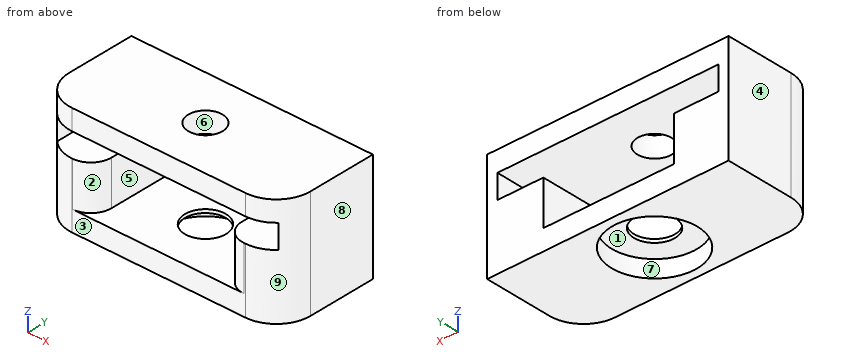
from build123d import *

# Parameters (mm, degrees)
SKETCH1_W           = 70.659898478
SKETCH1_H           = 30
BOSS_EXTRUDE1_DEPTH = 6
SKETCH2_R           = 5
CUT_EXTRUDE1_DEPTH  = 10
FILLET1_R           = 10
BOSS_EXTRUDE2_DEPTH = 7
BOSS_EXTRUDE3_DEPTH = 13
FILLET2_R           = 6
BOSS_EXTRUDE4_DEPTH = 6
SKETCH8_R           = 6
CUT_EXTRUDE2_DEPTH  = 30
SKETCH9_R           = 12.5
CUT_EXTRUDE3_DEPTH  = 5


with BuildPart() as part:
    # Sketch1 → Boss-Extrude1 (new body)
    with BuildSketch(Plane.XY):
        Rectangle(SKETCH1_W, SKETCH1_H)
    extrude(amount=BOSS_EXTRUDE1_DEPTH)

    # Sketch2 → Cut-Extrude1 (cut)
    with BuildSketch(Plane(origin=(0, 0, 0), x_dir=(-1, 0, 0), z_dir=(0, 0, -1))):
        Circle(SKETCH2_R)
    extrude(amount=-CUT_EXTRUDE1_DEPTH, mode=Mode.SUBTRACT)

    # Fillet1
    fillet1_edges = [part.edges().sort_by_distance(p)[0] for p in [
        (35.329949239, -15, 3),
        (-35.329949239, -15, 3),
    ]]
    fillet(fillet1_edges, radius=FILLET1_R)

    # Sketch4 → Boss-Extrude2 (add)
    with BuildSketch(Plane(origin=(0, 0, 0), x_dir=(-1, 0, 0), z_dir=(0, 0, -1))):
        with BuildLine():
            Line((-32.40101705, -12.071067812), (-32.316998846, 15))
            Line((-32.316998846, 15), (-35.329949239, 15))
            Line((-35.329949239, 15), (-35.329949239, -5))
            ThreePointArc((-35.329949239, -5), (-34.568744564, -8.826834324), (-32.40101705, -12.071067812))
        make_face()
        with BuildLine():
            Line((35.329949239, -5), (35.329949239, 15))
            Line((35.329949239, 15), (32.40101705, 15))
            Line((32.40101705, 15), (32.40101705, -12.071067812))
            ThreePointArc((32.40101705, -12.071067812), (34.568744564, -8.826834324), (35.329949239, -5))
        make_face()
    extrude(amount=BOSS_EXTRUDE2_DEPTH)

    # Sketch6 → Boss-Extrude3 (add)
    with BuildSketch(Plane(origin=(0, 0, -7), x_dir=(-1, 0, 0), z_dir=(0, 0, -1))):
        with BuildLine():
            Line((-18.889389891, 15), (-18.889389891, -15))
            Line((-18.889389891, -15), (-25.329949239, -15))
            ThreePointArc((-25.329949239, -15), (-32.40101705, -12.071067812), (-35.329949239, -5))
            Line((-35.329949239, -5), (-35.329949239, 15))
            Line((-35.329949239, 15), (-18.889389891, 15))
        make_face()
        with BuildLine():
            Line((19.317805732, 15), (19.317805732, -15))
            Line((19.317805732, -15), (25.329949239, -15))
            ThreePointArc((25.329949239, -15), (32.40101705, -12.071067812), (35.329949239, -5))
            Line((35.329949239, -5), (35.329949239, 15))
            Line((35.329949239, 15), (19.317805732, 15))
        make_face()
    extrude(amount=BOSS_EXTRUDE3_DEPTH)

    # Fillet2
    fillet2_edges = [part.edges().sort_by_distance(p)[0] for p in [
        (-19.317805732, -15, -13.5),
        (18.889389891, -15, -13.5),
    ]]
    fillet(fillet2_edges, radius=FILLET2_R)

    # Sketch7 → Boss-Extrude4 (add)
    with BuildSketch(Plane(origin=(0, 0, -20), x_dir=(-1, 0, 0), z_dir=(0, 0, -1))):
        with BuildLine():
            Line((-25.329949239, -15), (25.329949239, -15))
            ThreePointArc((25.329949239, -15), (32.40101705, -12.071067812), (35.329949239, -5))
            Line((35.329949239, -5), (35.329949239, 15))
            Line((35.329949239, 15), (-35.329949239, 15))
            Line((-35.329949239, 15), (-35.329949239, -5))
            ThreePointArc((-35.329949239, -5), (-32.40101705, -12.071067812), (-25.329949239, -15))
        make_face()
    extrude(amount=BOSS_EXTRUDE4_DEPTH)

    # Sketch8 → Cut-Extrude2 (cut)
    with BuildSketch(Plane.XY.offset(-20)):
        Circle(SKETCH8_R)
    extrude(amount=-CUT_EXTRUDE2_DEPTH, mode=Mode.SUBTRACT)

    # Sketch9 → Cut-Extrude3 (cut)
    with BuildSketch(Plane(origin=(0, 0, -26), x_dir=(-1, 0, 0), z_dir=(0, 0, -1))):
        Circle(SKETCH9_R)
    extrude(amount=-CUT_EXTRUDE3_DEPTH, mode=Mode.SUBTRACT)


solid = part.part
Verification items for the finished model (mm, model axes). Face numbers are marked on the shaded views. A direction names the side the tool comes from. Give positions to 0.01 mm unless a question says otherwise; leave off trailing zeros. Loops run counter-clockwise (first coordinate to the right, second up) from the corner with the lowest first, then second, coordinate; pieces in that order, holes last.
1) Draft check along Y on the marked faces 6, 7, 8 and 9. Enter one of: pulls with the +Y half, pulls with the -Y half, needs draft (parallel to the pull), parting line crosses it, or undercut.
2) Sectioned sample at C-C, the plane x = 0. Enter the section's corners in (y, z).
3) Sectioned sample at B-B, the plane z = 4. Enter the section's corners in (x, y), then the cut area to 3 significant figures.
4) Depth check by flat-ended pin: pin 1 Ø1.5 at (x, z) = (-28, -2) entering from +Y; pin 2 Ø9 at (x, y) = (-2, 1) entering from -Z; pin 3 Ø10 at (y, z) = (-11, -16.5) entering from -X. Enter the tip coordinate at first touch or a pass-through.
5) Thickness scan on line 1 along Z through (x, y) = (16.5, -1.5); line 2 along Z through (x, y) = (24, -4); line 3 along X through (y, z) = (8.5, -14). Record the ranges inside material, lowest first.
6) Sectioned sample at A-A, the plane x = 15.5. Enter the section's corners in (y, z).
7) Set-up check for the marked faces 1, 2, 3, 4 and 5: record each of +Z, -Z, +X, -X, +Y, -Y from which the full face is reachable in a straight line by a thin tool's end or side.
Answers:
1. face 6: undercut
1. face 7: undercut
1. face 8: needs draft
1. face 9: pulls with the -Y half
2. outline: (-15, -26) - (-12.5, -26) - (-12.5, -21) - (-6, -21) - (-6, -20) - (-15, -20) - close; (-15, 0) - (-5, 0) - (-5, 6) - (-15, 6) - close; (5, 0) - (15, 0) - (15, 6) - (5, 6) - close; (6, -21) - (12.5, -21) - (12.5, -26) - (15, -26) - (15, -20) - (6, -20) - close
3. outline: (-35.33, -5) arc R10 ccw to (-25.33, -15) - (25.33, -15) arc R10 ccw to (35.33, -5) - (35.33, 15) - (-35.33, 15) - close; hole circle Ø10 at (0, 0)
3. area: 2,000 mm2
4. pin 1: passes through
4. pin 2: stops at z = -21
4. pin 3: stops at x = -35.28
5. line 1: z = -26 to -20, 0 to 6
5. line 2: z = -26 to -7, 0 to 6
5. line 3: x = -35.33 to -19.32, 18.89 to 35.33
6. outline: (-15, -26) - (15, -26) - (15, -20) - (-15, -20) - close; (-15, 0) - (15, 0) - (15, 6) - (-15, 6) - close
7. face 1: -Z
7. face 2: -Y
7. face 3: +Z, -Z, +X, -X, -Y
7. face 4: +Z, -Z, -X, +Y, -Y
7. face 5: +Y, -Y
